from build123d import *

# Parameters (mm, degrees)
SKETCH1_W            = 133
SKETCH1_H            = 133
BOSS_EXTRUDE2_DEPTH  = 136
SKETCH2_W            = 133
SKETCH2_H            = 118
CUT_EXTRUDE1_DEPTH   = 136
BOSS_EXTRUDE3_DEPTH  = 10.5
SKETCH5_W            = 21
SKETCH5_H            = 3
BOSS_EXTRUDE4_DEPTH  = 23.5
SKETCH6_W            = 42
SKETCH6_H            = 17.2
CUT_EXTRUDE2_DEPTH   = 3
BOSS_EXTRUDE5_DEPTH  = 10.5
SKETCH8_W            = 21
SKETCH8_H            = 3
BOSS_EXTRUDE6_DEPTH  = 23.5
SKETCH9_W            = 42
SKETCH9_H            = 17.2
CUT_EXTRUDE3_DEPTH   = 3
SKETCH10_W           = 19.261488562
SKETCH10_H           = 133
BOSS_EXTRUDE7_DEPTH  = 5
SKETCH11_W           = 18.43727499
SKETCH11_H           = 133
BOSS_EXTRUDE8_DEPTH  = 5
SKETCH12_W           = 18.849381776
SKETCH12_H           = 146
BOSS_EXTRUDE9_DEPTH  = 12
SKETCH14_W           = 18.849381776
SKETCH14_H           = 146
BOSS_EXTRUDE10_DEPTH = 12
SKETCH17_R           = 1
CUT_EXTRUDE4_DEPTH   = 222.251553667
SKETCH20_W           = 133.244561713
SKETCH20_H           = 5
CUT_EXTRUDE10_DEPTH  = 19
SKETCH21_W           = 157
SKETCH21_H           = 120.66580897
CUT_EXTRUDE11_DEPTH  = 118
SKETCH22_W           = 186.174267818
SKETCH22_H           = 42.2523161
CUT_EXTRUDE12_DEPTH  = 118
SKETCH23_W           = 12
SKETCH23_H           = 25.33419103
CUT_EXTRUDE13_DEPTH  = 118
SKETCH24_W           = 12
SKETCH24_H           = 25.33419103
CUT_EXTRUDE14_DEPTH  = 118
SKETCH31_R           = 2.5
CUT_EXTRUDE21_DEPTH  = 118
SKETCH32_R           = 2.5
CUT_EXTRUDE22_DEPTH  = 118
SKETCH33_W           = 133
SKETCH33_H           = 5
CUT_EXTRUDE24_DEPTH  = 118
SKETCH34_R           = 2.5
CUT_EXTRUDE25_DEPTH  = 118
SKETCH35_R           = 4
CUT_EXTRUDE26_DEPTH  = 10


with BuildPart() as part:
    # Sketch1 → Boss-Extrude2 (new body)
    with BuildSketch(Plane(origin=(0, 0, 0), x_dir=(1, 0, 0), z_dir=(0, 1, 0))):
        Rectangle(SKETCH1_W, SKETCH1_H)
    extrude(amount=BOSS_EXTRUDE2_DEPTH)

    # Sketch2 → Cut-Extrude1 (cut)
    with BuildSketch(Plane.XY.offset(66.5)):
        with Locations((0, 68)):
            Rectangle(SKETCH2_W, SKETCH2_H)
    extrude(amount=-CUT_EXTRUDE1_DEPTH, mode=Mode.SUBTRACT)


with BuildPart() as cut_extrude1_piece_1:
    # of the separate pieces the step leaves, piece 1, a body of its own (cut_extrude1_pieces)
    add(part.part.solids().sort_by_distance((-66.5, 0, 66.5))[0])

    # Sketch4 → Boss-Extrude3 (add)
    with BuildSketch(Plane(origin=(0, 9, 0), x_dir=(1, 0, 0), z_dir=(0, 1, 0))):
        Polygon((22.75, -22.75), (43.75, -22.75), (46.25, -22.75), (46.25, -20.25), (20.25, -20.25), (20.25, -46.25), (46.25, -46.25), (46.25, -43.75), (43.75, -43.75), (22.75, -43.75), align=None)
        Polygon((22.75, 43.75), (43.75, 43.75), (46.25, 43.75), (46.25, 46.25), (20.25, 46.25), (20.25, 20.25), (46.25, 20.25), (46.25, 22.75), (43.75, 22.75), (22.75, 22.75), align=None)
    extrude(amount=BOSS_EXTRUDE3_DEPTH)

    # Sketch5 → Boss-Extrude4 (add)
    with BuildSketch(Plane(origin=(22.75, 0, 0), x_dir=(0, 0, -1), z_dir=(1, 0, 0))):
        with Locations((-33.25, 18)):
            Rectangle(SKETCH5_W, SKETCH5_H)
        with Locations((33.25, 18)):
            Rectangle(SKETCH5_W, SKETCH5_H)
    extrude(amount=BOSS_EXTRUDE4_DEPTH)

    # Sketch6 → Cut-Extrude2 (cut)
    with BuildSketch(Plane(origin=(0, 19.5, 0), x_dir=(1, 0, 0), z_dir=(0, 1, 0))):
        with Locations((46.25, -33.25)):
            Rectangle(SKETCH6_W, SKETCH6_H)
        with Locations((46.25, 33.25)):
            Rectangle(SKETCH6_W, SKETCH6_H)
    extrude(amount=-CUT_EXTRUDE2_DEPTH, mode=Mode.SUBTRACT)

    # Sketch10 → Boss-Extrude7 (add)
    with BuildSketch(Plane.XZ):
        Rectangle(SKETCH10_W, SKETCH10_H)
    extrude(amount=BOSS_EXTRUDE7_DEPTH)



with BuildPart() as cut_extrude1_piece_2:
    # of the separate pieces the step leaves, piece 2, a body of its own (cut_extrude1_pieces)
    add(part.part.solids().sort_by_distance((66.5, 127, 66.5))[0])

    # Sketch7 → Boss-Extrude5 (add)
    with BuildSketch(Plane.XZ.offset(-127)):
        Polygon((-43.75, 43.75), (-22.75, 43.75), (-22.75, 22.75), (-43.75, 22.75), (-46.25, 22.75), (-46.25, 20.25), (-20.25, 20.25), (-20.25, 46.25), (-46.25, 46.25), (-46.25, 43.75), align=None)
        Polygon((-43.75, -22.75), (-22.75, -22.75), (-22.75, -43.75), (-43.75, -43.75), (-46.25, -43.75), (-46.25, -46.25), (-20.25, -46.25), (-20.25, -20.25), (-46.25, -20.25), (-46.25, -22.75), align=None)
    extrude(amount=BOSS_EXTRUDE5_DEPTH)

    # Sketch8 → Boss-Extrude6 (add)
    with BuildSketch(Plane.ZY.offset(22.75)):
        with Locations((33.25, 118)):
            Rectangle(SKETCH8_W, SKETCH8_H)
        with Locations((-33.25, 118)):
            Rectangle(SKETCH8_W, SKETCH8_H)
    extrude(amount=BOSS_EXTRUDE6_DEPTH)

    # Sketch9 → Cut-Extrude3 (cut)
    with BuildSketch(Plane.XZ.offset(-116.5)):
        with Locations((-46.25, 33.25)):
            Rectangle(SKETCH9_W, SKETCH9_H)
        with Locations((-46.25, -33.25)):
            Rectangle(SKETCH9_W, SKETCH9_H)
    extrude(amount=-CUT_EXTRUDE3_DEPTH, mode=Mode.SUBTRACT)

    # Sketch11 → Boss-Extrude8 (add)
    with BuildSketch(Plane(origin=(0, 136, 0), x_dir=(1, 0, 0), z_dir=(0, 1, 0))):
        Rectangle(SKETCH11_W, SKETCH11_H)
    extrude(amount=BOSS_EXTRUDE8_DEPTH)


with BuildPart() as cut_extrude1_piece_1_1:
    add(cut_extrude1_piece_1.part)

    add(cut_extrude1_piece_2.part)  # Boss-Extrude9 merges Cut-Extrude1 piece 2
    # Sketch12 → Boss-Extrude9 (add)
    with BuildSketch(Plane(origin=(0, 0, -66.5), x_dir=(-1, 0, 0), z_dir=(0, 0, -1))):
        with Locations((-0.206053393, 68)):
            Rectangle(SKETCH12_W, SKETCH12_H)
    extrude(amount=BOSS_EXTRUDE9_DEPTH)

    # Sketch14 → Boss-Extrude10 (add)
    with BuildSketch(Plane.XY.offset(66.5)):
        with Locations((0.206053393, 68)):
            Rectangle(SKETCH14_W, SKETCH14_H)
    extrude(amount=BOSS_EXTRUDE10_DEPTH)

    # Sketch17 → Cut-Extrude4 (cut, through all)
    with BuildSketch(Plane.XY.offset(78.5)):
        with Locations((0.206053393, 68)):
            Circle(SKETCH17_R)
    extrude(amount=-CUT_EXTRUDE4_DEPTH, mode=Mode.SUBTRACT)

    # Sketch20 → Cut-Extrude10 (cut)
    with BuildSketch(Plane.ZY.offset(9.218637495)):
        with Locations((0.122280857, 138.5)):
            Rectangle(SKETCH20_W, SKETCH20_H)
    extrude(amount=-CUT_EXTRUDE10_DEPTH, mode=Mode.SUBTRACT)

    # Sketch21 → Cut-Extrude11 (cut)
    with BuildSketch(Plane.ZY.offset(9.218637495)):
        with Locations((0, 80.667095515)):
            Rectangle(SKETCH21_W, SKETCH21_H)
    extrude(amount=-CUT_EXTRUDE11_DEPTH, mode=Mode.SUBTRACT)


with BuildPart() as cut_extrude11_piece_1:
    # of the separate pieces the step leaves, piece 1, a body of its own (cut_extrude11_pieces)
    add(cut_extrude1_piece_1_1.part.solids().sort_by_distance((9.630744281, 20.33419103, 66.5))[0])

    # Sketch23 → Cut-Extrude13 (cut)
    with BuildSketch(Plane.ZY.offset(9.218637495)):
        with Locations((-72.5, 7.667095515)):
            Rectangle(SKETCH23_W, SKETCH23_H)
    extrude(amount=-CUT_EXTRUDE13_DEPTH, mode=Mode.SUBTRACT)

    # Sketch24 → Cut-Extrude14 (cut)
    with BuildSketch(Plane.ZY.offset(9.218637495)):
        with Locations((72.5, 7.667095515)):
            Rectangle(SKETCH24_W, SKETCH24_H)
    extrude(amount=-CUT_EXTRUDE14_DEPTH, mode=Mode.SUBTRACT)

    # Sketch31 → Cut-Extrude21 (cut)
    with BuildSketch(Plane.XZ.offset(5)):
        with Locations(Location((0, 59.499471122, 0), (0, 0, 270))):
            Circle(SKETCH31_R)
    extrude(amount=-CUT_EXTRUDE21_DEPTH, mode=Mode.SUBTRACT)

    # Sketch32 → Cut-Extrude22 (cut)
    with BuildSketch(Plane.XZ.offset(5)):
        with Locations(Location((0, -59.159797643, 0), (0, 0, 270))):
            Circle(SKETCH32_R)
    extrude(amount=-CUT_EXTRUDE22_DEPTH, mode=Mode.SUBTRACT)

    # Sketch33 → Cut-Extrude24 (cut)
    with BuildSketch(Plane.ZY.offset(9.630744281)):
        with Locations((0, -2.5)):
            Rectangle(SKETCH33_W, SKETCH33_H)
    extrude(amount=-CUT_EXTRUDE24_DEPTH, mode=Mode.SUBTRACT)

    # Sketch34 → Cut-Extrude25 (cut)
    with BuildSketch(Plane(origin=(0, 9, 0), x_dir=(1, 0, 0), z_dir=(0, 1, 0))):
        with Locations(Location((0, 0, 0), (0, 0, 270))):
            Circle(SKETCH34_R)
    extrude(amount=-CUT_EXTRUDE25_DEPTH, mode=Mode.SUBTRACT)

    # Sketch35 → Cut-Extrude26 (cut)
    with BuildSketch(Plane(origin=(0, 9, 0), x_dir=(1, 0, 0), z_dir=(0, 1, 0))):
        with Locations(Location((0, 0, 0), (0, 0, 270))):
            Circle(SKETCH35_R)
    extrude(amount=-CUT_EXTRUDE26_DEPTH, mode=Mode.SUBTRACT)


with BuildPart() as cut_extrude11_piece_2:
    # of the separate pieces the step leaves, piece 2, a body of its own (cut_extrude11_pieces)
    add(cut_extrude1_piece_1_1.part.solids().sort_by_distance((-9.218637495, 127, 66.5))[0])

    # Sketch22 → Cut-Extrude12 (cut)
    with BuildSketch(Plane.ZY.offset(66.5)):
        with Locations((20.706035589, 120.536042421)):
            Rectangle(SKETCH22_W, SKETCH22_H)
    extrude(amount=-CUT_EXTRUDE12_DEPTH, mode=Mode.SUBTRACT)


solid = cut_extrude11_piece_1.part
The model under review builds one solid part; all positions refer to its coordinate system, in mm. A direction names the side the tool comes from. Round coordinates to 2 decimals unless told otherwise and drop trailing zeros. Loops run counter-clockwise (first coordinate to the right, second up) from the corner with the lowest first, then second, coordinate; pieces in that order, holes last. Notation, with made-up numbers: (73, 65.5) -> (123, 65.5) arc R27 cw to (123, 101.5) -> close; hole circle Ø2 at (44.5, 84.5). An arc over 180 degrees is marked (long way). Return JSON: item names as keys, results as strings.
(1) For faces 3 (the flat face through (36, 18, 41.85)), 4 (the flat face through (35, 13, -22.75)), 5 (the flat face through (20.25, 14, 33)), 6 (the flat face through (46.25, 15, 22)), 7 (the flat face through (33, 14, -20.25)), list the 3-axis set-ups (+Z, -Z, +X, -X, +Y, -Y) from which the entire face can be reached by the end or side of a thin tool; tool diameter is ignored.
Solved:
{"face 3": "+X, +Y", "face 4": "+X", "face 5": "+Z, -Z, -X, +Y", "face 6": "+Z, -Z, +X, +Y", "face 7": "+X, -X, +Y"}
(2) The part is to be moulded in two halves that separate along Y. For faces 1 (the flat face through (46.25, 15, -22)), 2 (the flat face through (25, 16.5, 35)), say which applies: released by +Y, released by -Y, zero draft, split by the parting line, or undercut.
Solved:
{"face 1": "zero draft", "face 2": "undercut"}
(3) Add section D-D on x = 30. Write out the cut boundary in (y, z).
Solved:
{"outline": "(0, -66.5) -> (9, -66.5) -> (9, -46.25) -> (19.5, -46.25) -> (19.5, -41.85) -> (16.5, -41.85) -> (16.5, -43.75) -> (9, -43.75) -> (9, -22.75) -> (16.5, -22.75) -> (16.5, -24.65) -> (19.5, -24.65) -> (19.5, -20.25) -> (9, -20.25) -> (9, 20.25) -> (19.5, 20.25) -> (19.5, 24.65) -> (16.5, 24.65) -> (16.5, 22.75) -> (9, 22.75) -> (9, 43.75) -> (16.5, 43.75) -> (16.5, 41.85) -> (19.5, 41.85) -> (19.5, 46.25) -> (9, 46.25) -> (9, 66.5) -> (0, 66.5) -> close"}
(4) Add section B-B on z = 0. Write out the cut boundary in (x, y).
Solved:
{"outline": "(-66.5, 0) -> (-4, 0) -> (-4, 9) -> (-66.5, 9) -> close; (4, 0) -> (66.5, 0) -> (66.5, 9) -> (4, 9) -> close"}
(5) For pin 1 (6 mm diameter, centred on x = 37.5, y = 13, fed in from +Z); pin 2 (2 mm diameter, centred on y = 16, z = -23, fed in from +X); pin 3 (1.5 mm diameter, centred on x = 4.5, z = -18, fed in from +Y), all flat-tipped, find the tip position at first contact; note any pin that passes through.
Solved:
{"pin 1": "z = 46.25", "pin 2": "x = 46.25", "pin 3": "y = 9"}
(6) For line 1 (Y direction, x = 25, z = 31.5); line 2 (X direction, y = 5, z = 0); line 3 (Y direction, x = 54.5, z = 27), list the stretches that pass through material, from the lowest coordinate up.
Solved:
{"line 1": "0 to 9, 16.5 to 19.5", "line 2": "-66.5 to -4, 4 to 66.5", "line 3": "0 to 9"}
(7) Add section C-C on y = 12.5. Write out the cut boundary in (x, z), plus the area to 3 significant figures.
Solved:
{"outline": "(20.25, -46.25) -> (46.25, -46.25) -> (46.25, -43.75) -> (22.75, -43.75) -> (22.75, -22.75) -> (46.25, -22.75) -> (46.25, -20.25) -> (20.25, -20.25) -> close; (20.25, 20.25) -> (46.25, 20.25) -> (46.25, 22.75) -> (22.75, 22.75) -> (22.75, 43.75) -> (46.25, 43.75) -> (46.25, 46.25) -> (20.25, 46.25) -> close", "area": "365 mm2"}
(8) Add section A-A on x = 0. Write out the cut boundary in (y, z).
Solved:
{"outline": "(0, -66.5) -> (9, -66.5) -> (9, -61.66) -> (0, -61.66) -> close; (0, -56.66) -> (9, -56.66) -> (9, -4) -> (0, -4) -> close; (0, 4) -> (9, 4) -> (9, 57) -> (0, 57) -> close; (0, 62) -> (9, 62) -> (9, 66.5) -> (0, 66.5) -> close"}
